The figure shows three views and two pictorial views of one solid part (mm, origin at its lowest corner). Answer the questions. Coordinates: 2 decimals unless noted, no trailing zeros. Loops run counter-clockwise (first coordinate to the right, second up) from the corner with the lowest first, then second, coordinate; pieces in that order, holes last.
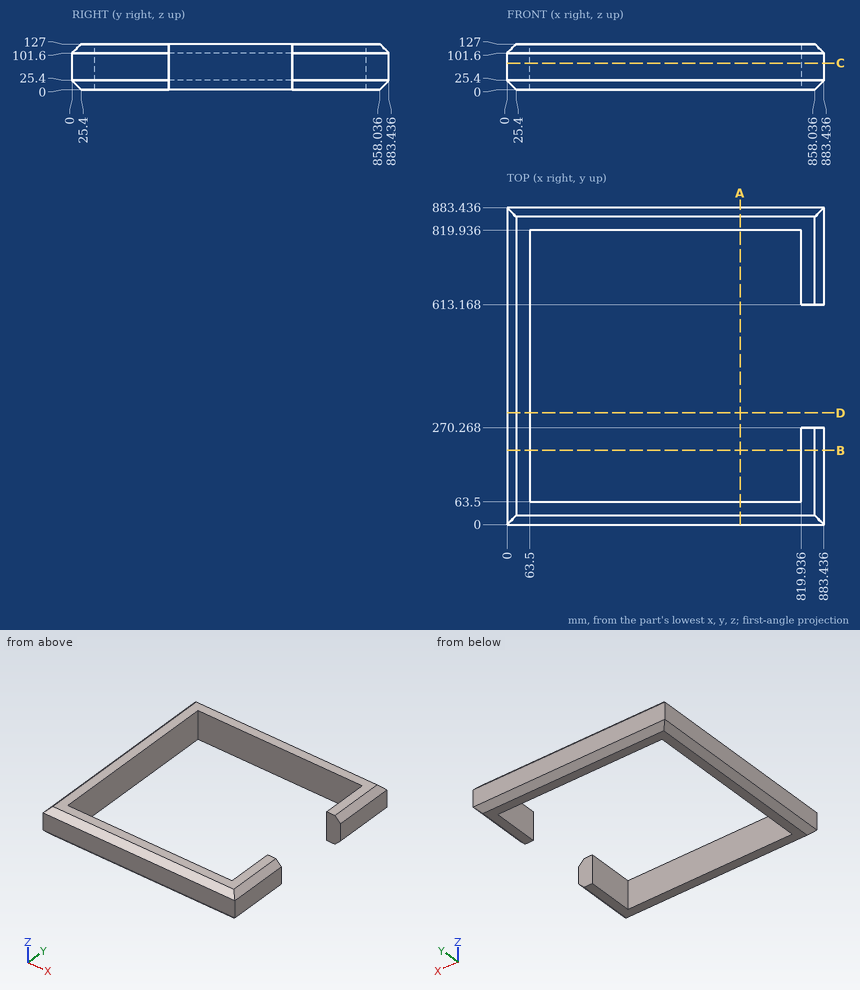
1. A cutting plane is placed at A-A, the plane x = 649.5. Give the vertices of the cut face in (y, z).
2. A cutting plane is placed at C-C, the plane z = 74. Give the vertices of the cut face in (x, y).
3. Straight lines are drawn through the part: probe 1 along X at (y, z) = (786.5, 68); probe 2 along Y at (x, z) = (846, 76.5). For each, find the intervals that lie inside material, in ascending order.
4. A cutting plane is placed at D-D, the plane y = 311. Give the vertices of the cut face in (x, z).
5. Each of these flat-tipped pins is pushed along its axis until it touches: P1, Ø4, axis at y = 480, z = 95, coming from the +X side; P2, Ø2, axis at x = 695.5, z = 17.5, coming from the +Y side. Where does it stop, or does it pass through?
Answers below:
1. outline: (0, 25.4) - (25.4, 0) - (63.5, 0) - (63.5, 127) - (25.4, 127) - (0, 101.6) - close; (819.94, 0) - (858.04, 0) - (883.44, 25.4) - (883.44, 101.6) - (858.04, 127) - (819.94, 127) - close
2. outline: (0, 0) - (883.44, 0) - (883.44, 270.27) - (819.94, 270.27) - (819.94, 63.5) - (63.5, 63.5) - (63.5, 819.94) - (819.94, 819.94) - (819.94, 613.17) - (883.44, 613.17) - (883.44, 883.44) - (0, 883.44) - close
3. probe 1: x = 0 to 63.5, 819.94 to 883.44
3. probe 2: y = 0 to 270.27, 613.17 to 883.44
4. outline: (0, 25.4) - (25.4, 0) - (63.5, 0) - (63.5, 127) - (25.4, 127) - (0, 101.6) - close
5. P1: stops at x = 63.5
5. P2: stops at y = 876.54
